Here's how the part is built. I have some questions about the finished solid (model axes, mm). Face numbers are marked on the shaded views. A direction names the side the tool comes from. Coordinates: 2 decimals unless noted, no trailing zeros. Write each loop counter-clockwise with the first axis right and the second up, starting at its lowest first coordinate (ties: lowest second). Pieces come first, ordered by that corner, then holes. Notation, with made-up numbers: M -38.5,61.25 L -12.5,61.25 A19 cw -12.5,83.25 Z; hole C 23.25,33 d1. An arc over 180 degrees is marked long. Use a Markdown table: item, result.
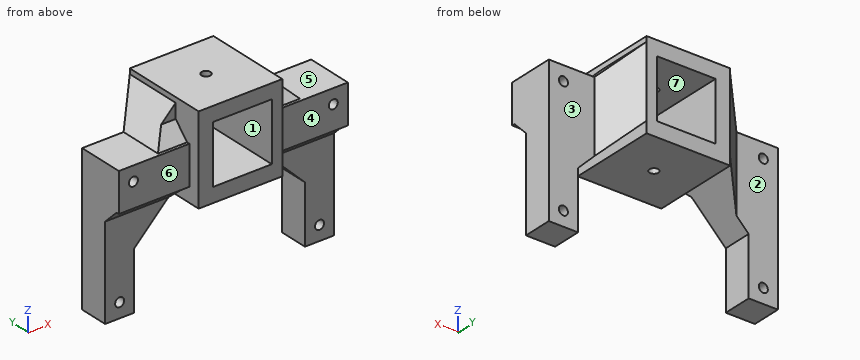
```python
from build123d import *

# Parameters (mm, degrees)
BOSS_EXTRUDE3_START = 180
SKETCH2_R           = 1.55
SKETCH2_W           = 25.630091621
SKETCH2_H           = 13.32
BOSS_EXTRUDE3_DEPTH = 10
BOSS_EXTRUDE4_START = 170
BOSS_EXTRUDE4_DEPTH = 30
CHAMFER1_SIZE       = 10
CHAMFER2_SIZE       = 10
SKETCH3_R           = 1.55
CUT_EXTRUDE1_DEPTH  = 43
BOSS_EXTRUDE5_START = 174
SKETCH2_5_W         = 25.630091621
SKETCH2_5_H         = 13.32
SKETCH2_5_R         = 1.55
BOSS_EXTRUDE5_DEPTH = 6.1
CHAMFER3_SIZE       = 5


with BuildPart() as part:
    # Sketch2 → Boss-Extrude3 (new body)
    # profile 1 of 8: a face of its own
    with BuildSketch(Plane(origin=(0, 0, 0), x_dir=(1, 0, 0), z_dir=(0, 1, 0)).offset(BOSS_EXTRUDE3_START)):
        Polygon((-39.3, 56.78), (-49.3, 56.78), (-49.3, 20.1), (-25.1, 20.1), (-25.1, 22.65), (-39.3, 36.85), align=None)
        with Locations(Location((-44.3, 51.78, 0), (0, 0, 270))):
            Circle(SKETCH2_R, mode=Mode.SUBTRACT)
    # profile 2 of 8: a face of its own
    with BuildSketch(Plane(origin=(0, 0, 0), x_dir=(1, 0, 0), z_dir=(0, 1, 0)).offset(BOSS_EXTRUDE3_START)):
        Polygon((-25.1, 20.1), (-49.3, 20.1), (-49.3, 6.78), (-40, 6.78), (-25.1, 6.78), align=None)
        with Locations(Location((-44.3, 11.78, 0), (0, 0, 270))):
            Circle(SKETCH2_R, mode=Mode.SUBTRACT)
    # profile 3 of 8: a face of its own
    with BuildSketch(Plane(origin=(0, 0, 0), x_dir=(1, 0, 0), z_dir=(0, 1, 0)).offset(BOSS_EXTRUDE3_START)):
        Polygon((-20.1, 6.78), (-25.1, 6.78), (-25.1, -5), (3.569908379, -5), (3.569908379, 6.78), (0, 6.78), (0, 0), (-20.1, 0), align=None)
    # profile 4 of 8: a face of its own
    with BuildSketch(Plane(origin=(0, 0, 0), x_dir=(1, 0, 0), z_dir=(0, 1, 0)).offset(BOSS_EXTRUDE3_START)):
        Polygon((-25.1, 22.65), (-25.1, 20.1), (-25.1, 6.78), (-20.1, 6.78), (-20.1, 20.1), (-22.55, 20.1), align=None)
    # profile 5 of 8: a face of its own
    with BuildSketch(Plane(origin=(0, 0, 0), x_dir=(1, 0, 0), z_dir=(0, 1, 0)).offset(BOSS_EXTRUDE3_START)):
        Polygon((-25.1, 25.1), (-25.1, 22.65), (-22.55, 20.1), (-20.1, 20.1), (0, 20.1), (2.45, 20.1), (3.569908379, 21.219908379), (3.569908379, 25.1), align=None)
    # profile 6 of 8: a face of its own
    with BuildSketch(Plane(origin=(0, 0, 0), x_dir=(1, 0, 0), z_dir=(0, 1, 0)).offset(BOSS_EXTRUDE3_START)):
        Polygon((0, 20.1), (0, 6.78), (3.569908379, 6.78), (3.569908379, 20.1), (3.569908379, 21.219908379), (2.45, 20.1), align=None)
    # profile 7 of 8: a face of its own
    with BuildSketch(Plane(origin=(0, 0, 0), x_dir=(1, 0, 0), z_dir=(0, 1, 0)).offset(BOSS_EXTRUDE3_START)):
        with Locations((16.38495419, 13.44)):
            Rectangle(SKETCH2_W, SKETCH2_H)
        with Locations(Location((24.2, 11.78, 0), (0, 0, 270))):
            Circle(SKETCH2_R, mode=Mode.SUBTRACT)
    # profile 8 of 8: a face of its own
    with BuildSketch(Plane(origin=(0, 0, 0), x_dir=(1, 0, 0), z_dir=(0, 1, 0)).offset(BOSS_EXTRUDE3_START)):
        Polygon((19.2, 36.85), (3.569908379, 21.219908379), (3.569908379, 20.1), (29.2, 20.1), (29.2, 56.78), (19.2, 56.78), align=None)
        with Locations(Location((24.2, 51.78, 0), (0, 0, 270))):
            Circle(SKETCH2_R, mode=Mode.SUBTRACT)
    extrude(amount=BOSS_EXTRUDE3_DEPTH)

    # Sketch2<3> → Boss-Extrude4 (add)
    with BuildSketch(Plane(origin=(0, 0, 0), x_dir=(1, 0, 0), z_dir=(0, 1, 0)).offset(BOSS_EXTRUDE4_START)):
        Polygon((-25.1, 22.65), (-25.1, 20.1), (-25.1, 6.78), (-20.1, 6.78), (-20.1, 20.1), (-22.55, 20.1), align=None)
        Polygon((-25.1, 25.1), (-25.1, 22.65), (-22.55, 20.1), (-20.1, 20.1), (0, 20.1), (2.45, 20.1), (3.569908379, 21.219908379), (3.569908379, 25.1), align=None)
        Polygon((0, 20.1), (0, 6.78), (3.569908379, 6.78), (3.569908379, 20.1), (3.569908379, 21.219908379), (2.45, 20.1), align=None)
        Polygon((-20.1, 6.78), (-25.1, 6.78), (-25.1, -5), (3.569908379, -5), (3.569908379, 6.78), (0, 6.78), (0, 0), (-20.1, 0), align=None)
    extrude(amount=BOSS_EXTRUDE4_DEPTH)

    # Chamfer1
    chamfer1_edges = [part.edges().sort_by_distance(p)[0] for p in [
        (-25.1, 190, -14.715),
        (3.569908379, 190, -13.999954189),
    ]]
    chamfer(chamfer1_edges, length=CHAMFER1_SIZE - 0.0001)  # a hair under: the kernel refuses the full size

    # Chamfer2
    chamfer2_edges = [part.edges().sort_by_distance(p)[0] for p in [
        (3.569908379, 189.99995, -6.78),
        (-25.1, 189.99995, -6.78),
    ]]
    chamfer(chamfer2_edges, length=CHAMFER2_SIZE)

    # Sketch3 → Cut-Extrude1 (cut)
    with BuildSketch(Plane(origin=(0, 0, -25.1), x_dir=(-1, 0, 0), z_dir=(0, 0, -1))):
        with Locations((10.765045811, 185)):
            Circle(SKETCH3_R)
    extrude(amount=-CUT_EXTRUDE1_DEPTH, mode=Mode.SUBTRACT)

    # Sketch2<5> → Boss-Extrude5 (add)
    # profile 1 of 2: a face of its own
    with BuildSketch(Plane(origin=(0, 0, 0), x_dir=(1, 0, 0), z_dir=(0, 1, 0)).offset(BOSS_EXTRUDE5_START)):
        with Locations((16.38495419, 13.44)):
            Rectangle(SKETCH2_5_W, SKETCH2_5_H)
        with Locations(Location((24.2, 11.78, 0), (0, 0, 270))):
            Circle(SKETCH2_5_R, mode=Mode.SUBTRACT)
    # profile 2 of 2: a face of its own
    with BuildSketch(Plane(origin=(0, 0, 0), x_dir=(1, 0, 0), z_dir=(0, 1, 0)).offset(BOSS_EXTRUDE5_START)):
        Polygon((-25.1, 20.1), (-49.3, 20.1), (-49.3, 6.78), (-40, 6.78), (-25.1, 6.78), align=None)
        with Locations(Location((-44.3, 11.78, 0), (0, 0, 270))):
            Circle(SKETCH2_5_R, mode=Mode.SUBTRACT)
    extrude(amount=BOSS_EXTRUDE5_DEPTH)

    # Chamfer3
    chamfer3_edges = [part.edges().sort_by_distance(p)[0] for p in [
        (16.384954189, 180, -20.1),
        (8.569908379, 180, -6.78),
        (-30.1, 180, -6.78),
        (-37.2, 180, -20.1),
    ]]
    chamfer(chamfer3_edges, length=CHAMFER3_SIZE)


solid = part.part
```
1. Suppose I cut it at B-B on x = -18.5. Write out the boundary of the cut face in (y, z), and give its area (3 significant figures).
Answers follow:
| item | result |
|---|---|
| outline | M 170,-25.1 L 200,-25.1 L 200,-20.1 L 170,-20.1 Z; M 170,0 L 200,0 L 200,5 L 170,5 Z |
| area | 300 mm2 |
2. Will these pins go through, and if not, where does the flat tip stop? pin 1 Ø1.1 at (x, y) = (-39.5, 174.5) entering from -Z; pin 2 Ø11 at (x, z) = (14, -42.5) entering from -Y; pin 3 Ø10.5 at (x, z) = (11.5, -11.5) entering from -Y.
Answers follow:
| item | result |
|---|---|
| pin 1 | stops at z = -20.15 |
| pin 2 | stops at y = 180 |
| pin 3 | stops at y = 174 |
3. We'd pull the mould along Z, two halves only. Please class the marked faces 5, 6 and 7: +Z half, -Z half, draft (parallel to the pull), parting line (faces both ways), or undercut.
Answers follow:
| item | result |
|---|---|
| face 5 | +Z half |
| face 6 | draft |
| face 7 | undercut |
4. Which directions (+Z, -Z, +X, -X, +Y, -Y) give clear straight access to the entire face, cutting with the end or side of a thin tool? Please do the marked faces 1, 2, 3 and 4.
Answers follow:
| item | result |
|---|---|
| face 1 | +Y, -Y |
| face 2 | +Z, -Z, -X, +Y |
| face 3 | +Z, -Z, +X, +Y |
| face 4 | +Z, -Z, +X, -Y |
5. Suppose I cut it at D-D on x = -44.3. Write out the boundary of the cut face in (y, z).
Answers follow:
| item | result |
|---|---|
| outline | M 174,-20.1 L 175,-20.1 L 180,-25.1 L 180,-50.23 L 190,-50.23 L 190,-13.33 L 174,-13.33 Z; M 174,-10.23 L 190,-10.23 L 190,-6.78 L 174,-6.78 Z; M 180,-56.78 L 190,-56.78 L 190,-53.33 L 180,-53.33 Z |
6. I need wall thicknesses on probe 1 along X at (y, z) = (184.5, -11.78); probe 2 along X at (y, z) = (185, -51.78); probe 3 along X at (y, z) = (172, -3). Which ranges of each line are inside material? Lowest first, please.
Answers follow:
| item | result |
|---|---|
| probe 1 | x = -49.3 to -45.85, -42.75 to -20.1, 0 to 22.65, 25.75 to 29.2 |
| probe 2 | x = -49.3 to -45.85, -42.75 to -39.3, 19.2 to 22.65, 25.75 to 29.2 |
| probe 3 | x = -25.1 to -20.1, 0 to 3.57 |
7. Suppose I cut it at A-A on y = 185. State how many separate pieces and enclosed holes the cut face has, and give its area (3 significant figures).
Answers follow:
| item | result |
|---|---|
| separate pieces | 2 |
| enclosed holes | 4 |
| area | 2,170 mm2 |
